Can you work these out from the model? Positions are in its coordinate system, mm. Face numbers are marked on the shaded views. A direction names the side the tool comes from. Coordinates: 2 decimals unless noted, no trailing zeros. Order: outer loops, then holes, each group sorted by start corner. A loop starts at its lowest first (then second) coordinate and runs counter-clockwise, first axis right, second up. Notation, with made-up numbers: (29.25, -29) -> (80.25, -29) arc R20 cw to (80.25, -3) -> close; hole circle Ø5 at (-19, 81.5). An arc over 180 degrees is marked (long way). Answer as CSV lines item,"result".
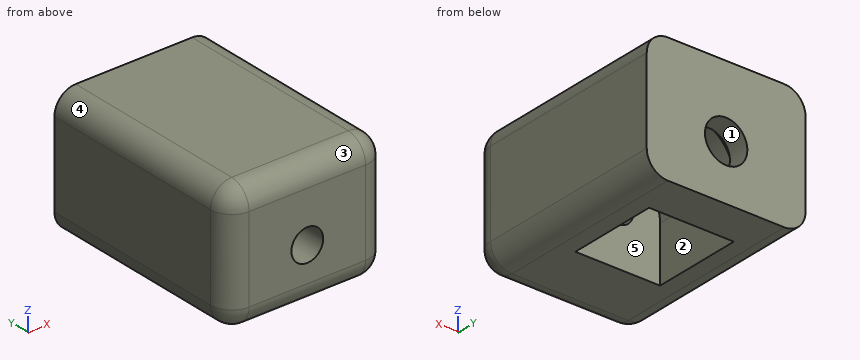
Autodesk Inventor part; units mm, degrees
ref_plane "YZ Plane" through (0, 0, 0) normal (1, 0, 0) x (0, 1, 0)
ref_plane "XZ Plane" through (0, 0, 0) normal (0, 1, 0) x (-1, 0, 0)
ref_plane "XY Plane" through (0, 0, 0) normal (0, 0, 1) x (1, 0, 0)
sketch "Sketch1" plane through (0, 0, 0) normal (0, 0, 1) x (1, 0, 0)
  line L0 (0, 0) -> (15, 0)
  line L1 (15, 0) -> (15, 20)
  line L2 (15, 20) -> (0, 20)
  line L3 (0, 20) -> (0, 0)
  dimension "d0" = 15
  dimension "d1" = 20
extrude "Extrusion1" add sketch "Sketch1" along normal blind 12
sketch "Sketch5" plane through (0, 0, 0) normal (0, 0, -1) x (-1, 0, 0)
  line L0 (0, 20) -> (0, 0)
  line L1 (-15, 20) -> (0, 20)
  line L2 (-11.5, 16) -> (-3.5, 16)
  line L3 (-3.5, 16) -> (-3.5, 7.5)
  line L4 (-3.5, 7.5) -> (-11.5, 7.5)
  line L5 (-11.5, 7.5) -> (-11.5, 16)
  dimension "d15" = 8
  dimension "d16" = 8.5
  dimension "d17" = 4
  dimension "d18" = 3.5
extrude "Extrusion4" cut sketch "Sketch5" against normal blind 9.237
fillet "Fillet1" radius 4 2 edges at (11.5, 11.75, 9.237) (3.5, 11.75, 9.237)
sketch "Sketch6" plane through (3.5, 16, 0) normal (0, -1, 0) x (1, 0, 0)
  arc A0 (8, 5.237) -> (0, 5.237) centre (4, 5.237) ccw
  circle A1 centre (4, 5.237) radius 2
  point P0 (-3.5, 0)
  dimension "d22" = 4
extrude "Extrusion5" cut sketch "Sketch6" against normal up to surface (4 mm away)
chamfer "Chamfer1" distance 2 angle 45 1 edges at (5.5, 16, 5.237)
sketch "Sketch7" plane through (3.5, 7.5, 0) normal (0, 1, 0) x (1, 0, 0)
  arc A0 (0, -5.237) -> (8, -5.237) centre (4, -5.237) ccw
  circle A1 centre (4, -5.237) radius 1.5
  point P0 (-3.5, 0)
  dimension "d28" = 3
extrude "Extrusion6" cut sketch "Sketch7" against normal up to surface (7.5 mm away)
fillet "Fillet2" radius 2 8 edges at (15, 0, 6) (0, 0, 6) (15, 10, 0) (15, 10, 12) (0, 10, 0) (7.5, 0, 0) (7.5, 0, 12) (0, 10, 12)
properties part number "PanelLedge" material "ABS Plastic"
Q1. If I drill on line 1 (Z direction, x = 7.5, y = 18.55); line 2 (Z direction, x = 7.5, y = 2.25); line 3 (X direction, y = 11.5, z = 3.5), over which ranges is the centre line in solid material (lowest first)?
Solution:
line 1,"0 to 3.24, 7.24 to 12"
line 2,"0 to 3.74, 6.74 to 12"
line 3,"0 to 3.5, 11.5 to 15"
Q2. Imagine slicing it at A-A (y = 2.5). List the corners of the cut face in (x, z) for me.
Solution:
outline,"(0, 2) arc R2 ccw to (2, 0) -> (13, 0) arc R2 ccw to (15, 2) -> (15, 10) arc R2 ccw to (13, 12) -> (2, 12) arc R2 ccw to (0, 10) -> close; hole circle Ø3 at (7.5, 5.24)"
Q3. We'd pull the mould along Y, two halves only. Please class the marked faces 1, 2 and 3: pulls with the +Y half, pulls with the -Y half, needs draft (parallel to the pull), parting line crosses it, or undercut.
Solution:
face 1,"needs draft"
face 2,"undercut"
face 3,"pulls with the -Y half"
Q4. Which directions (+Z, -Z, +X, -X, +Y, -Y) give clear straight access to the entire face, cutting with the end or side of a thin tool? Please do the marked faces 4 and 5.
Solution:
face 4,"+Z, -X, +Y, -Y"
face 5,"-Z"
Q5. Imagine slicing it at D-D (x = 6.5). Give the number of separate pieces and of enclosed holes in the cut face, and give its area (3 significant figures).
Solution:
separate pieces,"3"
enclosed holes,"0"
area,"126 mm2"
Q6. For P1, Ø4, axis at y = 11, z = 2.5, coming from the -X side; P2, Ø2.5, axis at x = 7.5, z = 5.237, coming from the -Y side, each with a flat end and sliding along its axis, tell me the tip position at first contact or that it passes through.
Solution:
P1,"x = 0"
P2,"through"
Q7. Imagine slicing it at C-C (z = 1). List the corners of the cut face in (x, y) for me, and give its area (3 significant figures).
Solution:
outline,"(0.27, 2) arc R1.73 ccw to (2, 0.27) -> (13, 0.27) arc R1.73 ccw to (14.73, 2) -> (14.73, 20) -> (0.27, 20) -> close; hole (3.5, 7.5) -> (11.5, 7.5) -> (11.5, 16) -> (3.5, 16) -> close"
area,"216 mm2"
